Source: CAD feature listing. Evaluate the final solid. Frame: model axes, mm. A direction names the side the tool comes from. Round coordinates to 2 decimals unless told otherwise and drop trailing zeros. Write each loop counter-clockwise with the first axis right and the second up, starting at its lowest first coordinate (ties: lowest second). Pieces come first, ordered by that corner, then holes. Notation, with made-up numbers: (4, 7) -> (24, 7) arc R13 ccw to (24, 19) -> close; hole circle Ø2 at (-16, 14.5). An arc over 180 degrees is marked (long way). Return JSON: item names as keys, results as strings. Group by question number.
Autodesk Inventor part; units mm, degrees
ref_plane "Work Plane2" through (11.25, 70.4, 1) normal (0, 1, 0) x (0, 0, 1)
ref_plane "Work Plane3" through (11.25, 42.7, 1) normal (0, -1, 0) x (1, 0, 0)
ref_plane "Work Plane4" through (11.925, 37.7, 1.675) normal (0, -1, 0) x (1, 0, 0)
ref_plane "Work Plane1" through (25.625, 84.2, 15.375) normal (0, 1, 0) x (0, 0, -1)
sketch "Sketch1" plane through (25.625, 84.2, 15.375) normal (0, 1, 0) x (0, 0, -1)
  line L0 (11.5, -1.5) -> (11, -1.5)
  line L1 (11, -1.5) -> (11, 1.5)
  line L2 (11, 1.5) -> (11.5, 1.5)
  line L3 (11.5, 1.5) -> (11.5, -1.5)
  line L4 (-12, -1.5) -> (-12, 1.5)
  line L5 (-12, 1.5) -> (-11.5, 1.5)
  line L6 (-11.5, 1.5) -> (-11.5, -1.5)
  line L7 (-11.5, -1.5) -> (-12, -1.5)
  circle A0 centre (0, 0) radius 5
  circle A1 centre (0, 0) radius 13.7
  line L8 (18.875, -15.375) -> (18.875, 116.625)
  line L9 (18.875, 116.625) -> (15.375, 116.625)
  line L10 (15.375, -15.375) -> (15.375, 116.625)
  line L11 (18.875, -15.375) -> (15.375, -15.375)
  line L12 (15.375, -15.375) -> (0, -15.375)
  line L13 (0, -15.375) -> (0, 15.375)
  line L14 (0, 15.375) -> (15.375, 15.375)
  line L15 (15.375, 15.375) -> (15.375, -15.375)
  circle A2 centre (12.125, 12.125) radius 3.25
  circle A3 centre (12.125, -12.125) radius 3.25
  line L16 (8.875, 15.375) -> (8.875, 10.4367)
  point P0 (15.375, 25.625)
  point P1 (0, -13.7)
  dimension "d2" = 15.375
  dimension "d3" = 15.375
  dimension "d4" = 6.5
  dimension "d5" = 6.5
ref_plane "Work Plane2" through (11.25, 70.4, 1) normal (0, 1, 0) x (0, 0, 1)
extrude "Extrusion1" add sketch "Sketch1" along normal blind 4.8 and the other way blind 13.8 contours A1 L16 A2 L10 A3 L12 L13 | L16 L14 A2 | A2 | A3 L10 L12 | A3 | L14 L10 A2
sketch "Sketch2" plane through (25.625, 70.4, 15.375) normal (0, -1, 0) x (1, 0, 0)
  arc A0 (-3.651, 5.9062) -> (-4.7619, 7.7035) centre (-4.2064, 6.8048) ccw
  arc A1 (-3.651, 5.9062) -> (-6.4477, 2.5768) centre (0, 0) ccw
  arc A2 (-8.4097, 3.3608) -> (-6.4477, 2.5768) centre (-7.4287, 2.9688) ccw
  arc A3 (-4.7619, 7.7035) -> (-8.4097, 3.3608) centre (0, 0) ccw
  arc A4 (6.4477, 2.5768) -> (8.4097, 3.3608) centre (7.4287, 2.9688) ccw
  arc A5 (6.4477, 2.5768) -> (3.651, 5.9062) centre (0, 0) ccw
  arc A6 (4.7619, 7.7035) -> (3.651, 5.9062) centre (4.2064, 6.8048) ccw
  arc A7 (8.4097, 3.3608) -> (4.7619, 7.7035) centre (0, 0) ccw
  arc A8 (-6.4563, -2.5553) -> (-8.4209, -3.3328) centre (-7.4386, -2.9441) ccw
  arc A9 (-6.4563, -2.5553) -> (-3.651, -5.9062) centre (0, 0) ccw
  arc A10 (-4.7619, -7.7035) -> (-3.651, -5.9062) centre (-4.2064, -6.8048) ccw
  arc A11 (-8.4209, -3.3328) -> (-4.7619, -7.7035) centre (0, 0) ccw
  arc A12 (3.651, -5.9062) -> (4.7619, -7.7035) centre (4.2064, -6.8048) ccw
  arc A13 (3.651, -5.9062) -> (6.4563, -2.5553) centre (0, 0) ccw
  arc A14 (8.4209, -3.3328) -> (6.4563, -2.5553) centre (7.4386, -2.9441) ccw
  arc A15 (4.7619, -7.7035) -> (8.4209, -3.3328) centre (0, 0) ccw
  circle A16 centre (10.65, 0.0124) radius 1.15
  circle A17 centre (0, 8) radius 1.0564
  circle A18 centre (0, -8) radius 1.0564
  circle A19 centre (0, 0) radius 5
  circle A20 centre (0, 0) radius 13.7
  line L0 (15.375, -18.875) -> (-116.625, -18.875)
  line L1 (-116.625, -18.875) -> (-116.625, -15.375)
  line L2 (15.375, -15.375) -> (-116.625, -15.375)
  line L3 (15.375, -18.875) -> (15.375, -15.375)
  line L4 (15.375, -15.375) -> (-15.375, -15.375)
  line L5 (-15.375, -15.375) -> (-15.375, 0)
  line L6 (-15.375, 0) -> (15.375, 0)
  line L7 (15.375, 0) -> (15.375, -15.375)
  circle A21 centre (0, 0) radius 14.375
  point P0 (-25.625, -15.375)
  point P1 (13.7, 0)
  point P2 (-13.7, 0)
  point P3 (-15.375, -15.375)
  point P4 (14.375, 0)
  point P5 (-14.375, 0)
  dimension "d10" = 15.375
  dimension "d11" = 15.375
ref_plane "Work Plane3" through (11.25, 42.7, 1) normal (0, -1, 0) x (1, 0, 0)
extrude "Extrusion2" add sketch "Sketch2" along normal up to surface (27.7 mm away) contours L6 L7 L2 L5 A21
sketch "Sketch3" plane through (25.625, 42.7, 15.375) normal (0, -1, 0) x (1, 0, 0)
  arc A0 (-3.651, 5.9062) -> (-4.7619, 7.7035) centre (-4.2064, 6.8048) ccw
  arc A1 (-3.651, 5.9062) -> (-6.4477, 2.5768) centre (0, 0) ccw
  arc A2 (-8.4097, 3.3608) -> (-6.4477, 2.5768) centre (-7.4287, 2.9688) ccw
  arc A3 (-4.7619, 7.7035) -> (-8.4097, 3.3608) centre (0, 0) ccw
  arc A4 (6.4477, 2.5768) -> (8.4097, 3.3608) centre (7.4287, 2.9688) ccw
  arc A5 (6.4477, 2.5768) -> (3.651, 5.9062) centre (0, 0) ccw
  arc A6 (4.7619, 7.7035) -> (3.651, 5.9062) centre (4.2064, 6.8048) ccw
  arc A7 (8.4097, 3.3608) -> (4.7619, 7.7035) centre (0, 0) ccw
  arc A8 (-6.4563, -2.5553) -> (-8.4209, -3.3328) centre (-7.4386, -2.9441) ccw
  arc A9 (-6.4563, -2.5553) -> (-3.651, -5.9062) centre (0, 0) ccw
  arc A10 (-4.7619, -7.7035) -> (-3.651, -5.9062) centre (-4.2064, -6.8048) ccw
  arc A11 (-8.4209, -3.3328) -> (-4.7619, -7.7035) centre (0, 0) ccw
  arc A12 (3.651, -5.9062) -> (4.7619, -7.7035) centre (4.2064, -6.8048) ccw
  arc A13 (3.651, -5.9062) -> (6.4563, -2.5553) centre (0, 0) ccw
  arc A14 (8.4209, -3.3328) -> (6.4563, -2.5553) centre (7.4386, -2.9441) ccw
  arc A15 (4.7619, -7.7035) -> (8.4209, -3.3328) centre (0, 0) ccw
  circle A16 centre (10.65, 0.0124) radius 1.15
  circle A17 centre (0, 8) radius 1.0564
  circle A18 centre (0, -8) radius 1.0564
  circle A19 centre (0, 0) radius 5
  circle A20 centre (0, 0) radius 13.7
  line L0 (15.375, -18.875) -> (-116.625, -18.875)
  line L1 (-116.625, -18.875) -> (-116.625, -15.375)
  line L2 (15.375, -15.375) -> (-116.625, -15.375)
  line L3 (15.375, -18.875) -> (15.375, -15.375)
  line L4 (15.375, 0) -> (15.375, -15.375)
  line L5 (15.375, -15.375) -> (-15.375, -15.375)
  line L6 (-15.375, -15.375) -> (-15.375, 0)
  line L7 (-15.375, 0) -> (15.375, 0)
  line L8 (15.375, 0) -> (15.375, -15.375)
  point P0 (-25.625, -15.375)
  point P1 (15.375, 0)
  point P2 (13.7, 0)
  point P3 (-13.7, 0)
  point P4 (-15.375, -15.375)
  dimension "d14" = 15.375
  dimension "d15" = 15.375
ref_plane "Work Plane4" through (11.925, 37.7, 1.675) normal (0, -1, 0) x (1, 0, 0)
extrude "Extrusion3" add sketch "Sketch3" along normal up to surface (5 mm away) contours L7 L4 L2 L6 A20
equation "\"d3\" = d2"
equation "\"d11\" = d10"
equation "\"d15\" = d14"
properties part number "motur_holder"
Item 1: Set-up query: faces 1 (the flat face through (11, 54, 15.375)), 2 (the flat face through (25.6, 42.7, 1.3)), 3 (the flat face through (11, 70.4, 10)). Return all of +Z, -Z, +X, -X, +Y, -Y with unobstructed straight access to the full face (end or side cutting, diameter ignored); none if empty.
Item 2: Cut plane D-D on z = 13.5. Output: boundary loops of the cut face in (x, y), and give its area (3 significant figures).
Item 3: First-contact query: pin 1 Ø2 at (x, z) = (26.5, 3) entering from -Y; pin 2 Ø4.5 at (x, z) = (13, 12.5) entering from +Y; pin 3 Ø5.5 at (x, y) = (13.5, 79) entering from +Z; pin 4 Ø2 at (x, y) = (33, 59) entering from +Z. Flat tips, straight axial feed; report the tip coordinate or a pass-through.
Item 4: Cut plane B-B on x = 17. Output: boundary loops of the cut face in (y, z) (3 decimals), and give its area (3 significant figures).
Item 5: Cut plane C-C on y = 72. Output: boundary loops of the cut face in (x, z) (3 decimals), and give its area (3 significant figures).
Item 6: Material intervals for probe 1 along Y at (x, z) = (25, 1.5); probe 2 along X at (y, z) = (61.5, 6.25); probe 3 along X at (y, z) = (50.5, 10.25), sorted ascending.
Item 7: Cut plane A-A on z = 8.5. Output: boundary loops of the cut face in (x, y).
Item 8: Pull-direction query (Y, two-part tool) for faces 4 (the flat face through (13, 80, 6.5)), 5 (the cylindrical face through (25.941, 56.744, 1.003)), 6 (the flat face through (25, 37.7, 1)); classes: +Y half, -Y half, draft (parallel to the pull), parting line (faces both ways), or undercut.
Here are the results:
{
 "1": {"face 1": "+Z, +X, -X, +Y, -Y", "face 2": "+Z", "face 3": "+Z, -X, +Y"},
 "2": {"outline": "(10.25, 37.7) -> (12.05, 37.7) -> (12.05, 42.7) -> (11.37, 42.7) -> (11.37, 70.4) -> (10.25, 70.4) -> close; (39.2, 37.7) -> (41, 37.7) -> (41, 89) -> (39.2, 89) -> (39.2, 70.4) -> (39.88, 70.4) -> (39.88, 42.7) -> (39.2, 42.7) -> close", "area": "114 mm^2"},
 "3": {"pin 1": "passes through", "pin 2": "stops at y = 70.4", "pin 3": "stops at z = 6.5", "pin 4": "stops at z = 3.69"},
 "4": {"outline": "(37.7, 0) -> (89, 0) -> (89, 4.731) -> (70.4, 4.731) -> (70.4, 3.875) -> (42.7, 3.875) -> (42.7, 4.731) -> (37.7, 4.731) -> close", "area": "219 mm^2"},
 "5": {"outline": "(10.25, 0) -> (41, 0) -> (41, 15.375) -> (39.325, 15.375) arc R13.7 cw to (15.188, 6.5) -> (10.25, 6.5) -> close", "area": "154 mm^2"},
 "6": {"probe 1": "y = 37.7 to 42.7, 70.4 to 89", "probe 2": "x = 10.25 to 14.52, 36.73 to 41", "probe 3": "x = 10.25 to 12.19, 39.06 to 41"},
 "7": {"outline": "(10.25, 37.7) -> (13.77, 37.7) -> (13.77, 42.7) -> (13, 42.7) -> (13, 70.4) -> (10.25, 70.4) -> close; (37.48, 37.7) -> (41, 37.7) -> (41, 89) -> (37.48, 89) -> (37.48, 70.4) -> (38.25, 70.4) -> (38.25, 42.7) -> (37.48, 42.7) -> close"},
 "8": {"face 4": "draft", "face 5": "undercut", "face 6": "-Y half"}
}
